```python
from build123d import *

# Parameters (mm, degrees)
SKETCH1_W           = 31.5
SKETCH1_H           = 20
SKETCH1_W_2         = 29.5
SKETCH1_H_2         = 18
EXTRUDE_THIN1_DEPTH = 8
BOSS_EXTRUDE1_START = 4
SKETCH2_W           = 31.5
SKETCH2_H           = 20
BOSS_EXTRUDE1_DEPTH = 1
SKETCH4_W           = 12.5
SKETCH4_H           = 20
BOSS_EXTRUDE2_DEPTH = 8
SKETCH5_R           = 1.35
CUT_EXTRUDE2_DEPTH  = 8
SKETCH12_W          = 1
SKETCH12_H          = 20
BOSS_EXTRUDE4_DEPTH = 22
BOSS_EXTRUDE6_START = 10.9
SKETCH3_R           = 1.5
BOSS_EXTRUDE6_DEPTH = 53.6


with BuildPart() as part:
    # Sketch1 → Extrude-Thin1 (new body)
    with BuildSketch(Plane.XY):
        with Locations((1.21969697, 10)):
            Rectangle(SKETCH1_W, SKETCH1_H)
        with Locations((1.21969697, 10)):
            Rectangle(SKETCH1_W_2, SKETCH1_H_2, mode=Mode.SUBTRACT)
    extrude(amount=EXTRUDE_THIN1_DEPTH)

    # Sketch2 → Boss-Extrude1 (add, symmetric)
    with BuildSketch(Plane.XY.offset(BOSS_EXTRUDE1_START)):
        with Locations((1.21969697, 10)):
            Rectangle(SKETCH2_W, SKETCH2_H)
    extrude(amount=BOSS_EXTRUDE1_DEPTH, both=True)

    # Sketch4 → Boss-Extrude2 (add)
    with BuildSketch(Plane.XY.offset(8)):
        with Locations((-8.28030303, 10)):
            Rectangle(SKETCH4_W, SKETCH4_H)
    extrude(amount=-BOSS_EXTRUDE2_DEPTH)

    # Sketch5 → Cut-Extrude2 (cut)
    with BuildSketch(Plane.XY.offset(8)):
        with Locations((-10.756674766, 5.895738268)):
            Circle(SKETCH5_R)
        with Locations((-5.502724413, 14.104261732)):
            Circle(SKETCH5_R)
    extrude(amount=-CUT_EXTRUDE2_DEPTH, mode=Mode.SUBTRACT)

    # Sketch12 → Boss-Extrude4 (add)
    with BuildSketch(Plane(origin=(0, 0, 0), x_dir=(-1, 0, 0), z_dir=(0, 0, -1))):
        with Locations((-16.46969697, 10)):
            Rectangle(SKETCH12_W, SKETCH12_H)
    extrude(amount=BOSS_EXTRUDE4_DEPTH)

    # Mirror5: part across plane


with BuildPart() as part_1:
    add(part.part)
    add(part.part.mirror(Plane.XY.offset(-11)))

    # Sketch3 → Boss-Extrude6 (add)
    with BuildSketch(Plane.XY.offset(5).offset(BOSS_EXTRUDE6_START)):
        with Locations((11.96969697, 10)):
            Circle(SKETCH3_R)
    extrude(amount=-BOSS_EXTRUDE6_DEPTH)


solid = part_1.part
```
Could you check a few things on this model? Use its own coordinates, in mm. A direction names the side the tool comes from. Round coordinates to 2 decimals unless told otherwise and drop trailing zeros. Order: outer loops, then holes, each group sorted by start corner. A loop starts at its lowest first (then second) coordinate and runs counter-clockwise, first axis right, second up. Notation, with made-up numbers: M -9.75,-5.5 L 18.25,-5.5 A18 cw 18.25,27.5 Z; hole C 49.5,65.5 d3. An arc over 180 degrees is marked long. One line per question, with ' | ' between items. Start each with the question number.
(1) Please list where these lines run through material, in increasing order: line 1 along Z through (x, y) = (-4.5, 19); line 2 along X through (y, z) = (6, 3.5); line 3 along X through (y, z) = (14, 6).
(2) For faces 1 (the face through (15.97, 10, 6)), 2 (the face through (-2.03, 10, 2)), 3 (the face through (7, 1, -28)), which set-ups out of +Z, -Z, +X, -X, +Y, -Y let a thin tool reach every point of the face, with its end or its side?
(3) Suppose I cut it at D-D on x = 15. List the corners of the cut face in (y, z) for me, then the cut area to 3 significant figures.
(4) Suppose I cut it at C-C on z = -12. List the corners of the cut face in (x, y) for me.
(5) For P1, Ø6, axis at x = -6.5, y = 10.5, coming from the -Z side; P2, Ø2, axis at x = -5.5, y = 14.1, coming from the -Z side; P3, Ø6, axis at y = 12, z = -14.5, coming from the -X side; P4, Ø6, axis at x = 5, y = 7, coming from the +Z side, each with a flat end and sliding along its axis, tell me the tip position at first contact or that it passes through.
(6) Thinking about a two-plate mould opening in X: for faces 4 (the face through (16.97, 10, -11)), 5 (the face through (-6, 12, 0)), 6 (the face through (10.47, 10.07, -32.28)), which applies, +X half, -X half, draft (parallel to the pull), parting line (faces both ways), or undercut?
(7) Suppose I cut it at A-A on x = -3. List the corners of the cut face in (y, z) for me.
Geometry results:
1) line 1: -30 to -22, 0 to 8 | line 2: -14.53 to -12.1, -9.41 to 16.97 | line 3: -14.53 to -6.85, -4.16 to -2.03, 15.97 to 16.97
2) face 1: +Z | face 2: none | face 3: -Z
3) outline: M 0,-30 L 1,-30 L 1,-27 L 19,-27 L 19,-30 L 20,-30 L 20,-22 L 19,-22 L 19,-25 L 1,-25 L 1,-22 L 0,-22 Z; M 0,0 L 1,0 L 1,3 L 19,3 L 19,0 L 20,0 L 20,8 L 19,8 L 19,5 L 1,5 L 1,8 L 0,8 Z | area: 104 mm²
4) outline: C 11.97,10 d3; M 15.97,0 L 16.97,0 L 16.97,20 L 15.97,20 Z
5) P1: z = -30 | P2: through | P3: x = 10.47 | P4: z = 5
6) face 4: +X half | face 5: draft | face 6: undercut
7) outline: M 0,-30 L 20,-30 L 20,-22 L 0,-22 Z; M 0,0 L 20,0 L 20,8 L 0,8 Z
